Could you check a few things on this model? Use its own coordinates, in mm. A direction names the side the tool comes from. Give positions to 0.01 mm unless a question says otherwise; leave off trailing zeros. Loops run counter-clockwise (first coordinate to the right, second up) from the corner with the lowest first, then second, coordinate; pieces in that order, holes last. Notation, with made-up numbers: M 73.25,33 L 89.25,33 A28 cw 89.25,61 Z; hole C -6.75,41.25 d7. An arc over 180 degrees is marked long. Answer in a Markdown table with one row per item. Add a question column.
```python
from build123d import *

# Parameters (mm, degrees)
BOSS_EXTRUDE1_START       = -11.2
BOSS_EXTRUDE1_DEPTH       = 15.2
BOSS_EXTRUDE1_START_2     = -11.30300619
BOSS_EXTRUDE1_2_OUTLINE_R = 9.525
BOSS_EXTRUDE1_2_DEPTH     = 0.10300619
BOSS_EXTRUDE1_START_3     = -1.5875
BOSS_EXTRUDE1_3_OUTLINE_R = 9.525
BOSS_EXTRUDE1_3_DEPTH     = 1.39699381
SKETCH2_R                 = 15
SKETCH2_R_2               = 7.854644271
BOSS_EXTRUDE2_DEPTH       = 1.5
SKETCH3_R                 = 15
SKETCH3_R_2               = 9.60106287
BOSS_EXTRUDE3_DEPTH       = 1.5
BOSS_EXTRUDE4_DEPTH       = 1.5
BOSS_EXTRUDE4_DEPTH_BACK  = 16.7
SKETCH5_R                 = 10.503090292
CUT_EXTRUDE1_DEPTH        = 28.950670833
FILLET1_R                 = 0.5
FILLET2_R                 = 0.5


with BuildPart() as part:
    # Boss-Extrude1: read off the stored shape, not the designer's step
    # Boss-Extrude1 outline → Boss-Extrude1 (new body)
    with BuildSketch(Plane(origin=(11.1125, 0, 0), x_dir=(0, 0, -1), z_dir=(1, 0, 0)).offset(BOSS_EXTRUDE1_START)):
        with BuildLine():
            ThreePointArc((12.692845514, 0.426230867), (11.294265748, 0.926615855), (9.809087715, 0.952242218))
            ThreePointArc((9.809087715, 0.952242218), (9.705477367, 1.71133752), (9.543213362, 2.4600906))
            ThreePointArc((9.543213362, 2.4600906), (10.930059468, 2.992132308), (12.073152809, 3.940682842))
            ThreePointArc((12.073152809, 3.940682842), (11.934096284, 4.34365582), (11.781593724, 4.741734842))
            ThreePointArc((11.781593724, 4.741734842), (10.296216892, 4.733600471), (8.891841322, 4.249720572))
            ThreePointArc((8.891841322, 4.249720572), (8.534853559, 4.9276), (8.126286635, 5.575700185))
            ThreePointArc((8.126286635, 5.575700185), (9.247526706, 6.549985156), (9.997259693, 7.832292041))
            ThreePointArc((9.997259693, 7.832292041), (9.728764428, 8.163402643), (9.449307854, 8.485315615))
            ThreePointArc((9.449307854, 8.485315615), (8.056292325, 7.96964301), (6.902107637, 7.034619905))
            ThreePointArc((6.902107637, 7.034619905), (6.334800451, 7.549521196), (5.729209809, 8.01879804))
            ThreePointArc((5.729209809, 8.01879804), (6.449605744, 9.317813127), (6.715549515, 10.779211228))
            ThreePointArc((6.715549515, 10.779211228), (6.35, 10.998522628), (5.977295999, 11.205442095))
            ThreePointArc((5.977295999, 11.205442095), (4.844660004, 10.244428982), (4.079877906, 8.971040258))
            ThreePointArc((4.079877906, 8.971040258), (3.370676917, 9.260858716), (2.641105726, 9.494710506))
            ThreePointArc((2.641105726, 9.494710506), (2.873767144, 10.961775319), (2.623844955, 12.425998457))
            ThreePointArc((2.623844955, 12.425998457), (2.205331856, 12.507058463), (1.784334031, 12.574026883))
            ThreePointArc((1.784334031, 12.574026883), (1.048690187, 11.283585627), (0.765554687, 9.825420757))
            ThreePointArc((0.765554687, 9.825420757), (0, 9.8552), (-0.765554687, 9.825420757))
            ThreePointArc((-0.765554687, 9.825420757), (-1.048690187, 11.283585627), (-1.784334031, 12.574026883))
            ThreePointArc((-1.784334031, 12.574026883), (-2.205331856, 12.507058463), (-2.623844955, 12.425998457))
            ThreePointArc((-2.623844955, 12.425998457), (-2.873767144, 10.961775319), (-2.641105726, 9.494710506))
            ThreePointArc((-2.641105726, 9.494710506), (-3.370676917, 9.260858716), (-4.079877906, 8.971040258))
            ThreePointArc((-4.079877906, 8.971040258), (-4.844660004, 10.244428982), (-5.977295999, 11.205442095))
            ThreePointArc((-5.977295999, 11.205442095), (-6.35, 10.998522628), (-6.715549515, 10.779211228))
            ThreePointArc((-6.715549515, 10.779211228), (-6.449605744, 9.317813127), (-5.729209809, 8.01879804))
            ThreePointArc((-5.729209809, 8.01879804), (-6.334800451, 7.549521196), (-6.902107637, 7.034619905))
            ThreePointArc((-6.902107637, 7.034619905), (-8.056292325, 7.96964301), (-9.449307854, 8.485315615))
            ThreePointArc((-9.449307854, 8.485315615), (-9.728764428, 8.163402643), (-9.997259693, 7.832292041))
            ThreePointArc((-9.997259693, 7.832292041), (-9.247526706, 6.549985156), (-8.126286635, 5.575700185))
            ThreePointArc((-8.126286635, 5.575700185), (-8.534853559, 4.9276), (-8.891841322, 4.249720572))
            ThreePointArc((-8.891841322, 4.249720572), (-10.296216892, 4.733600471), (-11.781593724, 4.741734842))
            ThreePointArc((-11.781593724, 4.741734842), (-11.934096284, 4.34365582), (-12.073152809, 3.940682842))
            ThreePointArc((-12.073152809, 3.940682842), (-10.930059468, 2.992132308), (-9.543213362, 2.4600906))
            ThreePointArc((-9.543213362, 2.4600906), (-9.705477367, 1.71133752), (-9.809087715, 0.952242218))
            ThreePointArc((-9.809087715, 0.952242218), (-11.294265748, 0.926615855), (-12.692845514, 0.426230867))
            ThreePointArc((-12.692845514, 0.426230867), (-12.7, 0), (-12.692845514, -0.426230867))
            ThreePointArc((-12.692845514, -0.426230867), (-11.294265748, -0.926615855), (-9.809087715, -0.952242218))
            ThreePointArc((-9.809087715, -0.952242218), (-9.705477367, -1.71133752), (-9.543213362, -2.4600906))
            ThreePointArc((-9.543213362, -2.4600906), (-10.930059468, -2.992132308), (-12.073152809, -3.940682842))
            ThreePointArc((-12.073152809, -3.940682842), (-11.934096284, -4.34365582), (-11.781593724, -4.741734842))
            ThreePointArc((-11.781593724, -4.741734842), (-10.296216892, -4.733600471), (-8.891841322, -4.249720572))
            ThreePointArc((-8.891841322, -4.249720572), (-8.534853559, -4.9276), (-8.126286635, -5.575700185))
            ThreePointArc((-8.126286635, -5.575700185), (-9.247526706, -6.549985156), (-9.997259693, -7.832292041))
            ThreePointArc((-9.997259693, -7.832292041), (-9.728764428, -8.163402643), (-9.449307854, -8.485315615))
            ThreePointArc((-9.449307854, -8.485315615), (-8.056292325, -7.96964301), (-6.902107637, -7.034619905))
            ThreePointArc((-6.902107637, -7.034619905), (-6.334800451, -7.549521196), (-5.729209809, -8.01879804))
            ThreePointArc((-5.729209809, -8.01879804), (-6.449605744, -9.317813127), (-6.715549515, -10.779211228))
            ThreePointArc((-6.715549515, -10.779211228), (-6.35, -10.998522628), (-5.977295999, -11.205442095))
            ThreePointArc((-5.977295999, -11.205442095), (-4.844660004, -10.244428982), (-4.079877906, -8.971040258))
            ThreePointArc((-4.079877906, -8.971040258), (-3.370676917, -9.260858716), (-2.641105726, -9.494710506))
            ThreePointArc((-2.641105726, -9.494710506), (-2.873767144, -10.961775319), (-2.623844955, -12.425998457))
            ThreePointArc((-2.623844955, -12.425998457), (-2.205331856, -12.507058463), (-1.784334031, -12.574026883))
            ThreePointArc((-1.784334031, -12.574026883), (-1.048690187, -11.283585627), (-0.765554687, -9.825420757))
            ThreePointArc((-0.765554687, -9.825420757), (0, -9.8552), (0.765554687, -9.825420757))
            ThreePointArc((0.765554687, -9.825420757), (1.048690187, -11.283585627), (1.784334031, -12.574026883))
            ThreePointArc((1.784334031, -12.574026883), (2.205331856, -12.507058463), (2.623844955, -12.425998457))
            ThreePointArc((2.623844955, -12.425998457), (2.873767144, -10.961775319), (2.641105726, -9.494710506))
            ThreePointArc((2.641105726, -9.494710506), (3.370676917, -9.260858716), (4.079877906, -8.971040258))
            ThreePointArc((4.079877906, -8.971040258), (4.844660004, -10.244428982), (5.977295999, -11.205442095))
            ThreePointArc((5.977295999, -11.205442095), (6.35, -10.998522628), (6.715549515, -10.779211228))
            ThreePointArc((6.715549515, -10.779211228), (6.449605744, -9.317813127), (5.729209809, -8.01879804))
            ThreePointArc((5.729209809, -8.01879804), (6.334800451, -7.549521196), (6.902107637, -7.034619905))
            ThreePointArc((6.902107637, -7.034619905), (8.056292325, -7.96964301), (9.449307854, -8.485315615))
            ThreePointArc((9.449307854, -8.485315615), (9.728764428, -8.163402643), (9.997259693, -7.832292041))
            ThreePointArc((9.997259693, -7.832292041), (9.247526706, -6.549985156), (8.126286635, -5.575700185))
            ThreePointArc((8.126286635, -5.575700185), (8.534853559, -4.9276), (8.891841322, -4.249720572))
            ThreePointArc((8.891841322, -4.249720572), (10.296216892, -4.733600471), (11.781593724, -4.741734842))
            ThreePointArc((11.781593724, -4.741734842), (11.934096284, -4.34365582), (12.073152809, -3.940682842))
            ThreePointArc((12.073152809, -3.940682842), (10.930059468, -2.992132308), (9.543213362, -2.4600906))
            ThreePointArc((9.543213362, -2.4600906), (9.705477367, -1.71133752), (9.809087715, -0.952242218))
            ThreePointArc((9.809087715, -0.952242218), (11.294265748, -0.926615855), (12.692845514, -0.426230867))
            ThreePointArc((12.692845514, -0.426230867), (12.7, 0), (12.692845514, 0.426230867))
        make_face()
        Polygon((3.666174209, 6.35), (7.332348419, 0), (3.666174209, -6.35), (-3.666174209, -6.35), (-7.332348419, 0), (-3.666174209, 6.35), align=None, mode=Mode.SUBTRACT)
    extrude(amount=BOSS_EXTRUDE1_DEPTH)

    # Boss-Extrude1 2 outline → Boss-Extrude1 2 (add)
    with BuildSketch(Plane(origin=(11.1125, 0, 0), x_dir=(0, 0, -1), z_dir=(1, 0, 0)).offset(BOSS_EXTRUDE1_START_2)):
        Circle(BOSS_EXTRUDE1_2_OUTLINE_R)
        Polygon((3.666174209, 6.35), (7.332348419, 0), (3.666174209, -6.35), (-3.666174209, -6.35), (-7.332348419, 0), (-3.666174209, 6.35), align=None, mode=Mode.SUBTRACT)
    extrude(amount=BOSS_EXTRUDE1_2_DEPTH)

    # Boss-Extrude1 3 outline → Boss-Extrude1 3 (add)
    with BuildSketch(Plane.YZ.offset(BOSS_EXTRUDE1_START_3)):
        Circle(BOSS_EXTRUDE1_3_OUTLINE_R)
        Polygon((6.35, -3.666174209), (0, -7.332348419), (-6.35, -3.666174209), (-6.35, 3.666174209), (0, 7.332348419), (6.35, 3.666174209), align=None, mode=Mode.SUBTRACT)
    extrude(amount=BOSS_EXTRUDE1_3_DEPTH)

    # Boss-Extrude1 4 outline → Boss-Extrude1 4 (revolve, cut)
    with BuildSketch(Plane.YX):
        Polygon((7.747, -1.5875), (6.34964944, -0.19014944), (6.34964944, -1.5875), align=None)
    revolve(axis=Axis((0, 0, 0), (1, 0, 0)), mode=Mode.SUBTRACT)

    # Sketch2 → Boss-Extrude2 (add)
    with BuildSketch(Plane(origin=(15.1125, 0, 0), x_dir=(0, 0, -1), z_dir=(1, 0, 0))):
        Circle(SKETCH2_R)
        Circle(SKETCH2_R_2, mode=Mode.SUBTRACT)
    extrude(amount=BOSS_EXTRUDE2_DEPTH)

    # Sketch3 → Boss-Extrude3 (add)
    with BuildSketch(Plane.ZY.offset(1.5875)):
        with Locations(Location((0, 0, 0), (0, 0, 180))):
            Circle(SKETCH3_R)
        Circle(SKETCH3_R_2, mode=Mode.SUBTRACT)
    extrude(amount=-BOSS_EXTRUDE3_DEPTH)

    # Sketch5 → Boss-Extrude4 (add, two sides: drawn at the far end of the back side and taken through both)
    with BuildSketch(Plane(origin=(15.1125, 0, 0), x_dir=(0, 0, -1), z_dir=(1, 0, 0)).offset(-BOSS_EXTRUDE4_DEPTH_BACK)):
        Circle(SKETCH5_R)
    extrude(amount=BOSS_EXTRUDE4_DEPTH + BOSS_EXTRUDE4_DEPTH_BACK)

    # Sketch4 → Cut-Extrude1 (cut, through all)
    with BuildSketch(Plane(origin=(16.6125, 0, 0), x_dir=(0, 0, -1), z_dir=(1, 0, 0))):
        Polygon((3.697448436, -6.531631373), (7.505282915, -0.063731412), (3.807834479, 6.467899962), (-3.697448436, 6.531631373), (-7.505282915, 0.063731412), (-3.807834479, -6.467899962), align=None)
    extrude(amount=-CUT_EXTRUDE1_DEPTH, mode=Mode.SUBTRACT)

    # Fillet1
    fillet1_edges = [part.edges().sort_by_distance(p)[0] for p in [
        (16.6125, -6.499765667, 0.055193021),
        (16.6125, -3.297681392, -5.601365676),
        (16.6125, 3.202084275, -5.656558697),
        (16.6125, 6.499765667, -0.055193021),
        (16.6125, 3.297681392, 5.601365676),
        (16.6125, -3.202084275, 5.656558697),
    ]]
    fillet(fillet1_edges, radius=FILLET1_R)

    # Fillet2
    fillet2_edges = [part.edges().sort_by_distance(p)[0] for p in [
        (-1.5875, -6.499765667, 0.055193021),
        (-1.5875, -3.202084275, 5.656558697),
        (-1.5875, 3.297681392, 5.601365676),
        (-1.5875, 6.499765667, -0.055193021),
        (-1.5875, 3.202084275, -5.656558697),
        (-1.5875, -3.297681392, -5.601365676),
    ]]
    fillet(fillet2_edges, radius=FILLET2_R)


solid = part.part
```
Item 1: Suppose I cut it at A-A (y = -9). List the corners of the cut face in (x, z) for me.
Item 2: For faces 4 (the face through (7.406, -12.506, 2.211)), 5 (the face through (7.406, -8.053, -6.742)), 6 (the face through (7.406, 6.793, -9.436)), 7 (the face through (7.41, 10.47, 5.05)), which set-ups out of +Z, -Z, +X, -X, +Y, -Y let a thin tool reach every point of the face, with its end or its side?
Item 3: If we mould it in two halves opening along X, with no side actions, what happens to faces 1 (the face through (7.406, -4.775, -10.601)), 2 (the face through (16.46, -3.32, 5.75)), 3 (the face through (7.6, 3.3, 5.6))? For each: +X half, -X half, draft (parallel to the pull), parting line (faces both ways), or undercut.
Item 4: For P1, Ø10, axis at x = 4, y = 9.5, coming from the -Z side; P2, Ø10, axis at x = 6, y = -0.5, coming from the -Z side; P3, Ø2, axis at x = 13.5, y = -3.5, coming from the -Z side, each with a flat end and sliding along its axis, tell me the tip position at first contact or that it passes through.
Item 5: I need wall thicknesses on L1, parallel to X at y = -6, z = 11.25; L2, parallel to Y at x = 4.25, z = 11.75; L3, parallel to Y at x = 5.5, z = -4.75. Which ranges of each line are inside material? Lowest first, please.
Values found:
| question | item | result |
|---|---|---|
| 1 | outline | M -1.59,-12 L -0.09,-12 L -0.09,-6.32 L 15.11,-6.32 L 15.11,-12 L 16.61,-12 L 16.61,12 L 15.11,12 L 15.11,6.32 L -0.09,6.32 L -0.09,12 L -1.59,12 Z |
| 2 | face 4 | +Z, -Y |
| 2 | face 5 | none |
| 2 | face 6 | -Z |
| 2 | face 7 | +Y |
| 3 | face 1 | undercut |
| 3 | face 2 | +X half |
| 3 | face 3 | draft |
| 4 | P1 | z = -13.46 |
| 4 | P2 | z = -12.7 |
| 4 | P3 | z = -12.07 |
| 5 | L1 | -1.59 to -0.09, 15.11 to 16.61 |
| 5 | L2 | -4.75 to -3.6, -0.82 to 0.82, 3.6 to 4.75 |
| 5 | L3 | -10.13 to -4.74, 4.8 to 10.13 |
